Model file for the job. Use its own axes, mm. A direction names the side the tool comes from. Give positions to 0.01 mm unless a question says otherwise; leave off trailing zeros. Answer in a Markdown table with one row per item. Add a question column.
Autodesk Inventor part; units mm, degrees
ref_plane "Work Plane3" through (19.7324, 0, 119.8626) normal (0, 0.7071, -0.7071) x (-1, 0, 0)
ref_plane "YZ Plane" through (0, 0, 0) normal (1, 0, 0) x (0, 1, 0)
ref_plane "XZ Plane" through (0, 0, 0) normal (0, 1, 0) x (-1, 0, 0)
sketch "Sketch1" plane through (0, 0, 0) normal (0, 0, 1) x (1, 0, 0)
  circle A0 centre (0, 0) radius 31.75
  dimension "d0" = 63.5
extrude "Extrusion1" add sketch "Sketch1" along normal blind 174.625
sketch "Sketch2" plane through (0, 0, 174.625) normal (0, 0, 1) x (1, 0, 0)
  circle A0 centre (0, 0) radius 31.75
  circle A1 centre (0, 0) radius 26.2509
  dimension "d3" = 52.5018
extrude "Extrusion2" cut sketch "Sketch2" against normal blind 174.625 contours A1
sketch "Sketch3" plane through (0, 0, 174.625) normal (0, 0, 1) x (1, 0, 0)
  circle A0 centre (0, 0) radius 26.2509
  circle A1 centre (0, 0) radius 31.75
  circle A2 centre (0, 0) radius 30.1625
  dimension "d7" = 60.325
extrude "Extrusion3" cut sketch "Sketch3" against normal blind 38.1 contours A2
sketch "Sketch4" plane through (0, 0, 0) normal (0, 0, -1) x (-1, 0, 0)
  circle A0 centre (0, 0) radius 26.2509
  circle A1 centre (0, 0) radius 31.75
  circle A2 centre (0, 0) radius 30.1625
  dimension "d11" = 60.325
extrude "Extrusion4" cut sketch "Sketch4" against normal blind 38.1 contours A2
sketch "Sketch5" plane through (0, 0, 0) normal (0, 0, -1) x (-1, 0, 0)
  circle A0 centre (0, 0) radius 30.1625
  circle A1 centre (0, 0) radius 31.75
  point P0 (0, 31.75)
ref_plane "Work Plane2" through (0, 0, 0) normal (0, 1, 0) x (-1, 0, 0)
ref_plane "Work Plane1" through (0, 31.75, 0) normal (0, 1, 0) x (-1, 0, 0)
sketch "Sketch6" plane through (0, 0, 0) normal (0, 1, 0) x (-1, 0, 0)
  line L0 (-19.7324, 119.8626) -> (17.0407, 119.8626) construction
  line L1 (-30.1625, 174.625) -> (30.1625, 174.625) construction
  point P0 (0, 0)
  dimension "d15" = 54.7624
ref_plane "Work Plane3" through (19.7324, 0, 119.8626) normal (0, 0.7071, -0.7071) x (-1, 0, 0)
sketch "Sketch7" plane through (19.7324, 0, 119.8626) normal (0, 0.7071, -0.7071) x (-1, 0, 0)
  circle A0 centre (19.7324, -0.166) radius 31.75
  point P0 (19.7324, -84.7557)
  dimension "d18" = 63.5
extrude "Extrusion5" add sketch "Sketch7" along normal blind 119.38
sketch "Sketch8" plane through (0, 84.297, 35.3308) normal (0, 0.7071, -0.7071) x (-1, 0, 0)
  circle A0 centre (0, 0) radius 31.75
  circle A1 centre (0, 0) radius 30.1625
  point P0 (0, -84.5897)
  dimension "d21" = 60.325
extrude "Extrusion6" cut sketch "Sketch8" against normal blind 35.56 contours A1
sketch "Sketch9" plane through (0, 59.1523, 60.4755) normal (0, 0.7071, -0.7071) x (-1, 0, 0)
  circle A0 centre (0, 0) radius 30.1625
  circle A1 centre (0, 0) radius 26.162
  point P0 (0, -84.5897)
  dimension "d24" = 52.324
extrude "Extrusion8" cut sketch "Sketch9" against normal blind 35.56 contours A1
properties part number "sup-wye" material "PVC-Piping"
Item 1: Saw through at D-D on z = 18.5. Give the number of separate pieces and of enclosed holes in the cut face, plus the area to 3 significant figures.
Item 2: Pin check, flat tips, straight feed: pin 1 Ø8 at (x, y) = (-9, 87.5) entering from -Z; pin 2 Ø3 at (x, y) = (-18.5, 17.5) entering from +Z; pin 3 Ø18 at (x, y) = (1.5, -7.5) entering from +Z. Stop position of each tip, or through.
Item 3: Wall check: line 1 (Y direction, x = 0, z = 146); line 2 (Y direction, x = -17, z = 93); line 3 (X direction, y = 0, z = 77). Give the ranges that are in metal, low to high.
Item 4: Which spindle directions (+Z, -Z, +X, -X, +Y, -Y) get a long thin tool onto all of the face, cutting with end or side? Do faces 4 (the cylindrical face through (0.323, 24.504, 140.023)), 5 (the flat face through (0.366, 34.265, 85.881)), 6 (the flat face through (9, 25, 38.1)), 7 (the flat face through (-28.074, 76.087, 27.121)). Say none if no direction does.
Item 5: Two-plate mould, pull along Z, no slides. Class faces 1 (the flat face through (9.078, 76.629, 77.955)), 2 (the cylindrical face through (6.88, 72.84, 90.62)), 3 (the cylindrical face through (30.133, 1.326, 18.783)): pulls with the +Z half, pulls with the -Z half, needs draft (parallel to the pull), parting line crosses it, or undercut.
Evaluation:
| question | item | result |
|---|---|---|
| 1 | separate pieces | 2 |
| 1 | enclosed holes | 1 |
| 1 | area | 405 mm2 |
| 2 | pin 1 | stops at z = 68.38 |
| 2 | pin 2 | stops at z = 138.48 |
| 2 | pin 3 | stops at z = 121.36 |
| 3 | line 1 | y = -31.75 to -30.16, 30.16 to 31.75 |
| 3 | line 2 | y = -26.82 to -20, -11.29 to 41.38, 54.75 to 64.55 |
| 3 | line 3 | x = -31.75 to -26.25, -9.97 to 9.97, 26.25 to 31.75 |
| 4 | face 4 | +Z |
| 4 | face 5 | none |
| 4 | face 6 | -Z |
| 4 | face 7 | -Z, +X, -X, +Y |
| 5 | face 1 | undercut |
| 5 | face 2 | parting line crosses it |
| 5 | face 3 | needs draft |
